For this review, use the dimensioned drawing (mm, ordinates from the lowest corner) and the shaded views. A direction names the side the tool comes from. Round coordinates to 2 decimals unless told otherwise and drop trailing zeros. Loops run counter-clockwise (first coordinate to the right, second up) from the corner with the lowest first, then second, coordinate; pieces in that order, holes last. Notation, with made-up numbers: (-1, 51) - (37, 51) arc R13 ccw to (37, 60) - close; hole circle Ø3 at (82.5, -30.75). An arc over 180 degrees is marked (long way). One line per question, with ' | ' between items. Start each with the question number.
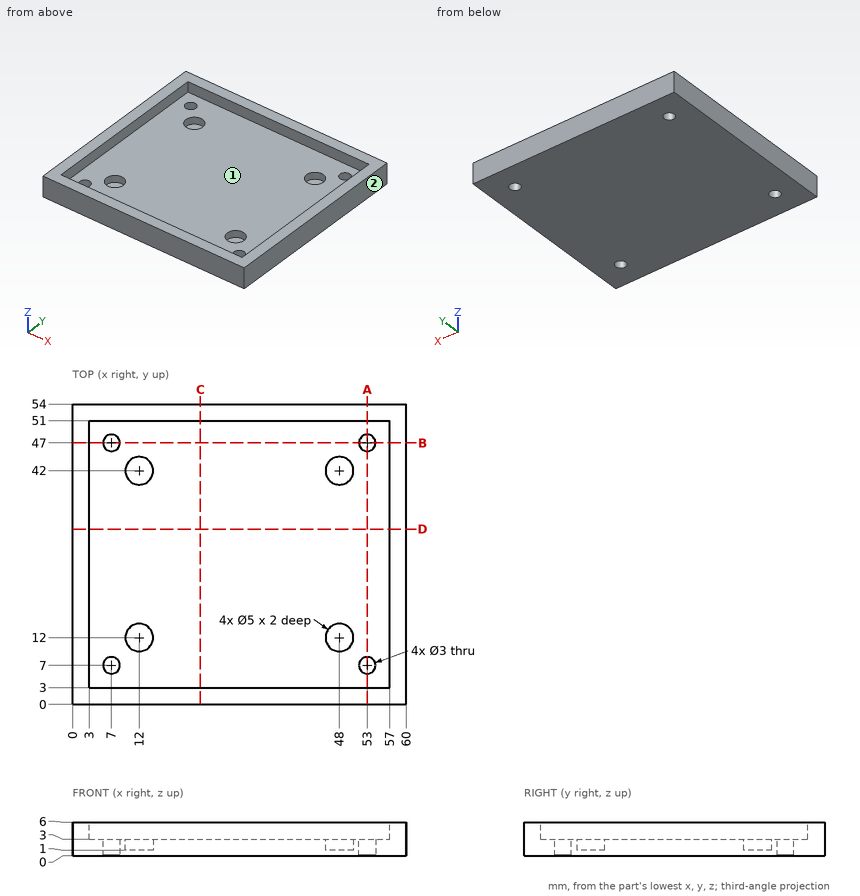
1. Take a section at D-D, the plane y = 31.5. Give the boundary of the cut face in (x, z), then the cut area to 3 significant figures.
2. Take a section at A-A, the plane x = 53. Give the boundary of the cut face in (y, z).
3. Machinability: for the marked faces 1 and 2, which of the approach directions +Z, -Z, +X, -X, +Y, -Y give a long, thin tool a straight path to every point of the face, cutting with its end or side? Answer none if there is none.
4. Take a section at C-C, the plane x = 23. Give the boundary of the cut face in (y, z).
5. Clearance check with flat-ended pins moving along their axes: P1, Ø10, axis at x = 48, y = 15, coming from the +Z side; P2, Ø5, axis at x = 51.5, y = 46.5, coming from the -Z side; P3, Ø1.5, axis at x = 48.5, y = 42.5, coming from the +Z side. State where each tip first meets the part, or that it passes through.
6. To check wall thickness, follow line 1 along Y through (x, z) = (53, 0.75); line 2 along X through (y, z) = (10.5, 4.4); line 3 along Y through (x, z) = (12, 2.2). State the ranges of each line that lie inside material, in increasing order.
7. Take a section at B-B, the plane y = 47. Give the boundary of the cut face in (x, z), then the cut area to 3 significant figures.
Answer list:
1) outline: (0, 0) - (60, 0) - (60, 6) - (57, 6) - (57, 3) - (3, 3) - (3, 6) - (0, 6) - close | area: 198 mm²
2) outline: (0, 0) - (5.5, 0) - (5.5, 3) - (3, 3) - (3, 6) - (0, 6) - close; (8.5, 0) - (45.5, 0) - (45.5, 3) - (8.5, 3) - close; (48.5, 0) - (54, 0) - (54, 6) - (51, 6) - (51, 3) - (48.5, 3) - close
3) face 1: +Z | face 2: +Z, -Z, +X, +Y, -Y
4) outline: (0, 0) - (54, 0) - (54, 6) - (51, 6) - (51, 3) - (3, 3) - (3, 6) - (0, 6) - close
5) P1: stops at z = 3 | P2: stops at z = 0 | P3: stops at z = 1
6) line 1: y = 0 to 5.5, 8.5 to 45.5, 48.5 to 54 | line 2: x = 0 to 3, 57 to 60 | line 3: y = 0 to 9.5, 14.5 to 39.5, 44.5 to 54
7) outline: (0, 0) - (5.5, 0) - (5.5, 3) - (3, 3) - (3, 6) - (0, 6) - close; (8.5, 0) - (51.5, 0) - (51.5, 3) - (8.5, 3) - close; (54.5, 0) - (60, 0) - (60, 6) - (57, 6) - (57, 3) - (54.5, 3) - close | area: 180 mm²
